from build123d import *

# Parameters (mm, degrees)
SKETCH_R        = 50
PAD_DEPTH       = 42
SKETCH001_R     = 48
POCKET_DEPTH    = 40
PAD001_DEPTH    = 40
SKETCH005_W     = 9.3
SKETCH005_H     = 11.3
POCKET001_DEPTH = 10
SKETCH006_W     = 6
SKETCH006_H     = 9
PAD004_DEPTH    = 10
POCKET002_DEPTH = 8
SKETCH009_R     = 5
PAD006_DEPTH    = 4
SKETCH011_W     = 0.5
SKETCH011_H     = 9.3
PAD007_DEPTH    = 0.5
SKETCH012_R     = 5
PAD008_DEPTH    = 3
POCKET004_DEPTH = 2
SKETCH014_R     = 1.5
POCKET005_DEPTH = 4
POCKET006_DEPTH = 2
SKETCH015_R     = 1.5
POCKET007_DEPTH = 5
SKETCH016_R     = 2
POCKET008_DEPTH = 5.8
POCKET009_DEPTH = 5


with BuildPart() as part:
    # Sketch → Pad (new body)
    with BuildSketch(Plane.XY):
        Circle(SKETCH_R)
    extrude(amount=PAD_DEPTH)

    # Sketch001 (on DatumPlane) → Pocket (cut)
    with BuildSketch(Plane.XY.offset(42)):
        Circle(SKETCH001_R)
    extrude(amount=-POCKET_DEPTH, mode=Mode.SUBTRACT)

    # Sketch002 (on DatumPlane) → Pad001 (join)
    with BuildSketch(Plane.XY.offset(42)):
        with BuildLine():
            ThreePointArc((-38.205841, 17.44459), (-32.908965, 19), (-34.210379, 24.364934))
            Line((-34.210379, 24.364934), (-40.104744, 28.153322))
            ThreePointArc((-40.104744, 28.153322), (-42.435245, 24.5), (-44.433864, 20.655066))
            Line((-38.205841, 17.44459), (-44.433864, 20.655066))
        make_face()
        with BuildLine():
            ThreePointArc((3.995462, -41.809524), (0, -38), (-3.995462, -41.809524))
            Line((-3.995462, -41.809524), (-4.32912, -48.808388))
            ThreePointArc((-4.32912, -48.808388), (0, -49), (4.32912, -48.808388))
            Line((3.995462, -41.809524), (4.32912, -48.808388))
        make_face()
        with BuildLine():
            ThreePointArc((34.210379, 24.364934), (32.908965, 19), (38.205841, 17.44459))
            Line((38.205841, 17.44459), (44.433864, 20.655066))
            ThreePointArc((44.433864, 20.655066), (42.435245, 24.5), (40.104744, 28.153322))
            Line((34.210379, 24.364934), (40.104744, 28.153322))
        make_face()
    extrude(amount=-PAD001_DEPTH)

    # Sketch005 (on DatumPlane) → Pocket001 (cut)
    with BuildSketch(Plane.YZ.offset(50)):
        with Locations((0, 7.65)):
            Rectangle(SKETCH005_W, SKETCH005_H)
    extrude(amount=-POCKET001_DEPTH, mode=Mode.SUBTRACT)

    # Sketch006 (on DatumPlane) → Pad004 (join)
    with BuildSketch(Plane.XY.offset(2)):
        with Locations((40, 0)):
            Rectangle(SKETCH006_W, SKETCH006_H)
    extrude(amount=PAD004_DEPTH)

    # Sketch007 (on Face18 of Pad004) → Pocket002 (cut)
    with BuildSketch(Plane.YZ.offset(43)):
        with BuildLine():
            ThreePointArc((-3.99875, 6.6), (0, 2.7), (3.99875, 6.6))
            Line((5.575286, 6.6), (3.99875, 6.6))
            Line((5.575286, 15.969053), (5.575286, 6.6))
            Line((-6.906295, 15.969053), (5.575286, 15.969053))
            Line((-6.906295, 6.6), (-6.906295, 15.969053))
            Line((-3.99875, 6.6), (-6.906295, 6.6))
        make_face()
    extrude(amount=-POCKET002_DEPTH, mode=Mode.SUBTRACT)

    # Sketch009 (on DatumPlane) → Pad006 (join)
    with BuildSketch(Plane.XY.offset(2)):
        with Locations((-22.75, 32.75)):
            Circle(SKETCH009_R)
        with Locations((22.75, 32.75)):
            Circle(SKETCH009_R)
        with Locations((22.75, -32.75)):
            Circle(SKETCH009_R)
        with Locations((-22.75, -32.75)):
            Circle(SKETCH009_R)
    extrude(amount=PAD006_DEPTH)

    # Sketch011 (on DatumPlane) → Pad007 (join)
    with BuildSketch(Plane.XY.offset(2)):
        with Locations((49.533305, 0)):
            Rectangle(SKETCH011_W, SKETCH011_H)
    extrude(amount=PAD007_DEPTH)

    # Sketch012 (on DatumPlane) → Pad008 (join)
    with BuildSketch(Plane.XY.offset(2)):
        with Locations((37.35, -11.5)):
            Circle(SKETCH012_R)
    pad008 = extrude(amount=PAD008_DEPTH)

    # Sketch013 (on Face47 of Pad008) → Pocket004 (cut)
    with BuildSketch(Plane.XY.offset(5)):
        Polygon((39.925, -12.986677), (39.925, -10.013323), (37.35, -8.526646), (34.775, -10.013323), (34.775, -12.986677), (37.35, -14.473354), align=None)
    pocket004 = extrude(amount=-POCKET004_DEPTH, mode=Mode.SUBTRACT)

    # Sketch014 (on Face47 of Pocket004) → Pocket005 (cut)
    with BuildSketch(Plane.XY.offset(5)):
        with Locations((37.35, -11.5)):
            Circle(SKETCH014_R)
    pocket005 = extrude(amount=-POCKET005_DEPTH, mode=Mode.SUBTRACT)

    # Sketch010 (on DatumPlane) → Pocket006 (cut)
    with BuildSketch(Plane.XY.offset(6)):
        Polygon((-20.175, 31.263323), (-20.175, 34.236677), (-22.75, 35.723354), (-25.325, 34.236677), (-25.325, 31.263323), (-22.75, 29.776646), align=None)
        Polygon((25.325, -34.236677), (25.325, -31.263323), (22.75, -29.776646), (20.175, -31.263323), (20.175, -34.236677), (22.75, -35.723354), align=None)
        Polygon((22.75, 35.723354), (20.175, 34.236677), (20.175, 31.263323), (22.75, 29.776646), (25.325, 31.263323), (25.325, 34.236677), align=None)
        Polygon((-20.175, -31.263323), (-22.75, -29.776646), (-25.325, -31.263323), (-25.325, -34.236677), (-22.75, -35.723354), (-20.175, -34.236677), align=None)
    extrude(amount=-POCKET006_DEPTH, mode=Mode.SUBTRACT)

    # Sketch015 (on DatumPlane) → Pocket007 (cut)
    with BuildSketch(Plane.XY.offset(6)):
        with Locations((-22.75, 32.75)):
            Circle(SKETCH015_R)
        with Locations((22.75, 32.75)):
            Circle(SKETCH015_R)
        with Locations((22.7, -32.75)):
            Circle(SKETCH015_R)
        with Locations((-22.75, -32.75)):
            Circle(SKETCH015_R)
    extrude(amount=-POCKET007_DEPTH, mode=Mode.SUBTRACT)

    # Sketch016 (on DatumPlane) → Pocket008 (cut)
    with BuildSketch(Plane.XY.offset(42)):
        with Locations((-36.373067, 21)):
            Circle(SKETCH016_R)
        with Locations((36.373067, 21)):
            Circle(SKETCH016_R)
        with Locations((0, -42)):
            Circle(SKETCH016_R)
    extrude(amount=-POCKET008_DEPTH, mode=Mode.SUBTRACT)

    # Mirrored: Pad008, Pocket004, Pocket005 across Sketch012 H_Axis
    add(pad008.mirror(Plane(origin=(0, 0, 2), x_dir=(0, 0, 1), z_dir=(0, 1, 0))))
    add(pocket004.mirror(Plane(origin=(0, 0, 2), x_dir=(0, 0, 1), z_dir=(0, 1, 0))), mode=Mode.SUBTRACT)
    add(pocket005.mirror(Plane(origin=(0, 0, 2), x_dir=(0, 0, 1), z_dir=(0, 1, 0))), mode=Mode.SUBTRACT)

    # Sketch018 (on DatumPlane) → Pocket009 (cut)
    with BuildSketch(Plane(origin=(-18.476599, -46.460901, 42), x_dir=(0.929218, -0.369532, 0), z_dir=(-0.369532, -0.929218, 0))):
        with BuildLine():
            add(Edge.make_bspline(
                [(0, -28.745076), (7.727306, -28.745076), (3.863653, -17.127462), (0, -5.509849), (-3.863653, -17.127462), (-7.727306, -28.745076), (0, -28.745076)],
                knots=[0, 0, 0, 2.094395, 2.094395, 4.18879, 4.18879, 6.283185, 6.283185, 6.283185], degree=2, weights=[1, 0.5, 1, 0.5, 1, 0.5, 1]))
        make_face()
    extrude(amount=-POCKET009_DEPTH, mode=Mode.SUBTRACT)


solid = part.part
The listing builds one solid part. Answer for the finished solid, in the listing's coordinates (mm). Give positions to 0.01 mm unless a question says otherwise; leave off trailing zeros. Order: outer loops, then holes, each group sorted by start corner. A loop starts at its lowest first (then second) coordinate and runs counter-clockwise, first axis right, second up. Notation, with made-up numbers: (29.5, 25) -> (73.5, 25) arc R20 cw to (73.5, 38) -> close; hole circle Ø10 at (58.25, -7). An arc over 180 degrees is marked (long way). Put each result on its own line as item: value.
Item 1: A cutting plane is placed at B-B on x = 0. Give the vertices of the cut face in (y, z).
Established:
outline: (-50, 0) -> (50, 0) -> (50, 42) -> (48, 42) -> (48, 2) -> (-38, 2) -> (-38, 42) -> (-40, 42) -> (-40, 36.2) -> (-44, 36.2) -> (-44, 42) -> (-50, 42) -> close
Item 2: A cutting plane is placed at A-A on y = 0. Give the vertices of the cut face in (x, z).
Established:
outline: (-50, 0) -> (50, 0) -> (50, 2) -> (49.78, 2) -> (49.78, 2.5) -> (49.28, 2.5) -> (49.28, 2) -> (43, 2) -> (43, 2.7) -> (37, 2.7) -> (37, 2) -> (-48, 2) -> (-48, 42) -> (-50, 42) -> close; (48, 13.3) -> (50, 13.3) -> (50, 42) -> (48, 42) -> close
Item 3: A cutting plane is placed at C-C on z = 8. Give the vertices of the cut face in (x, y), plus the area to 3 significant figures.
Established:
outline: (-43.54, 20.2) -> (-38.21, 17.44) arc R4 ccw to (-34.21, 24.36) -> (-39.26, 27.61) arc R48 cw to (39.26, 27.61) -> (34.21, 24.36) arc R4 ccw to (38.21, 17.44) -> (43.54, 20.2) arc R48 cw to (47.77, 4.65) -> (49.78, 4.65) arc R50 ccw (long way) to (49.78, -4.65) -> (47.77, -4.65) arc R48 cw to (4.28, -47.81) -> (4, -41.81) arc R4 ccw to (-4, -41.81) -> (-4.28, -47.81) arc R48 cw to start
area: 820 mm^2
Item 4: Given P1, Ø2, axis at y = 32.5, z = 4.5, coming from the -X side; P2, Ø1.5, axis at x = -22.5, y = -32.5, coming from the +Z side; P3, Ø3, axis at y = 16, z = 4.5, coming from the +X side, each flat-ended and moving along its own axis, determine where each tip first touches the part or whether it passes through.
Established:
P1: stops at x = -38.83
P2: stops at z = 1
P3: stops at x = 47.85
Item 5: Straight lines are drawn through the part: line 1 (Y direction, x = 33, z = 29); line 2 (Z direction, x = 3, y = 43.5); line 3 (Y direction, x = -8, z = 33). For each, find the intervals that lie inside material, in ascending order.
Established:
line 1: y = -37.56 to -34.86, 18.85 to 23.15, 34.86 to 37.56
line 2: z = 0 to 2
line 3: y = -49.36 to -47.33, 47.33 to 49.36
Item 6: A cutting plane is placed at D-D on y = 41. Give the vertices of the cut face in (x, z).
Established:
outline: (-28.62, 0) -> (28.62, 0) -> (28.62, 42) -> (24.96, 42) -> (24.96, 2) -> (-24.96, 2) -> (-24.96, 42) -> (-28.62, 42) -> close
Item 7: For a pull along X with two mould halves and no side action, classify faces 1 (the face through (-4.136, -44.767, 22.28)), 2 (the face through (-34, 19, 42)), 3 (the face through (47.69, 15.02, 20.71)) as released by +X, released by -X, zero draft, split by the parting line, or undercut.
Established:
face 1: undercut
face 2: zero draft
face 3: split by the parting line
